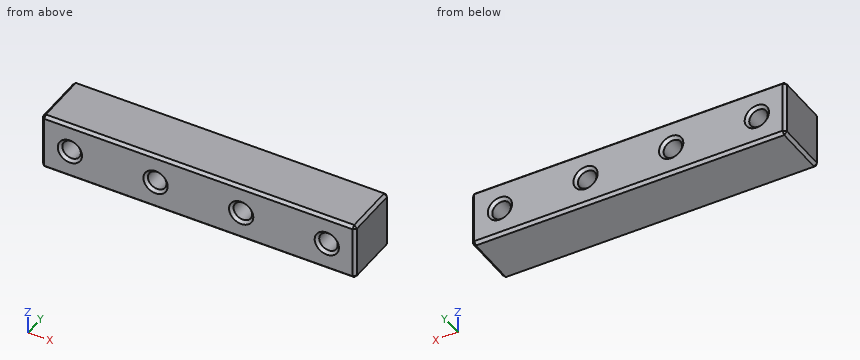
```python
from build123d import *

# Parameters (mm, degrees)
SKETCH1_W           = 110
SKETCH1_H           = 20
SKETCH1_R           = 3.25
BOSS_EXTRUDE1_DEPTH = 20
CHAMFER1_SIZE       = 1


with BuildPart() as part:
    # Sketch1 → Boss-Extrude1 (new body)
    with BuildSketch(Plane(origin=(0, 0, 0), x_dir=(1, 0, 0), z_dir=(0, 1, 0))):
        Rectangle(SKETCH1_W, SKETCH1_H)
        with Locations(Location((-45, 0, 0), (0, 0, 270))):
            Circle(SKETCH1_R, mode=Mode.SUBTRACT)
        with Locations(Location((-15, 0, 0), (0, 0, 270))):
            Circle(SKETCH1_R, mode=Mode.SUBTRACT)
        with Locations(Location((15, 0, 0), (0, 0, 270))):
            Circle(SKETCH1_R, mode=Mode.SUBTRACT)
        with Locations(Location((45, 0, 0), (0, 0, 270))):
            Circle(SKETCH1_R, mode=Mode.SUBTRACT)
    extrude(amount=BOSS_EXTRUDE1_DEPTH)

    # Chamfer1
    chamfer1_edges = [part.edges().sort_by_distance(p)[0] for p in [
        (-45, 0, -3.25),
        (-45, 20, -3.25),
        (-55, 20, 0),
        (-15, 0, -3.25),
        (-15, 20, -3.25),
        (0, 20, 10),
        (15, 0, -3.25),
        (15, 20, -3.25),
        (45, 0, -3.25),
        (45, 20, -3.25),
        (55, 20, 0),
        (0, 0, 10),
        (-55, 0, 0),
        (0, 0, -10),
        (55, 0, 0),
        (55, 10, 10),
        (-55, 10, 10),
        (-55, 10, -10),
        (55, 10, -10),
        (0, 20, -10),
    ]]
    chamfer(chamfer1_edges, length=CHAMFER1_SIZE)


solid = part.part
```
Source: CAD feature listing. Evaluate the final solid. Frame: model axes, mm. Give positions to 0.01 mm unless a question says otherwise; leave off trailing zeros. Loops run counter-clockwise (first coordinate to the right, second up) from the corner with the lowest first, then second, coordinate; pieces in that order, holes last. Notation, with made-up numbers: (70, 71) -> (87, 71) arc R31 cw to (87, 108) -> close; hole circle Ø7 at (11.5, -14.75). An arc over 180 degrees is marked (long way). Put each result on its own line as item: value. Start each with the question number.
1) Material intervals for probe 1 along X at (y, z) = (5, 0); probe 2 along X at (y, z) = (17.5, -1); probe 3 along Z at (x, y) = (-16, 4.25), sorted ascending.
2) Cut plane B-B (x = -45). Return loops of the section in (y, z), then the cut area to 3 significant figures.
3) Cut plane C-C (z = 0). State how many separate pieces and enclosed holes the cut face has, then the cut area to 3 significant figures.
4) Cut plane A-A (y = 15.25). Return loops of the section in (x, z).
5) Contact query for a flat-ended pin moving along its axis: P1, Ø7.5, axis at x = 45, z = 0, coming from the +Y side. Output: stop coordinate, or through.
Results are:
1. probe 1: x = -55 to -48.25, -41.75 to -18.25, -11.75 to 11.75, 18.25 to 41.75, 48.25 to 55
1. probe 2: x = -55 to -48.09, -41.91 to -18.09, -11.91 to 11.91, 18.09 to 41.91, 48.09 to 55
1. probe 3: z = -10 to -3.09, 3.09 to 10
2. outline: (0, -9) -> (1, -10) -> (19, -10) -> (20, -9) -> (20, -4.25) -> (19, -3.25) -> (1, -3.25) -> (0, -4.25) -> close; (0, 4.25) -> (1, 3.25) -> (19, 3.25) -> (20, 4.25) -> (20, 9) -> (19, 10) -> (1, 10) -> (0, 9) -> close
2. area: 266 mm2
3. separate pieces: 5
3. enclosed holes: 0
3. area: 1,670 mm2
4. outline: (-55, -9) -> (-54, -10) -> (54, -10) -> (55, -9) -> (55, 9) -> (54, 10) -> (-54, 10) -> (-55, 9) -> close; hole circle Ø6.5 at (-45, 0); hole circle Ø6.5 at (-15, 0); hole circle Ø6.5 at (15, 0); hole circle Ø6.5 at (45, 0)
5. P1: stops at y = 19.5
